Could you check a few things on this model? Use its own coordinates, in mm. A direction names the side the tool comes from. Give positions to 0.01 mm unless a question says otherwise; leave off trailing zeros. Loops run counter-clockwise (first coordinate to the right, second up) from the corner with the lowest first, then second, coordinate; pieces in that order, holes last. Notation, with made-up numbers: (-7, 57.25) -> (42, 57.25) arc R24 cw to (42, 79.25) -> close; hole circle Ø1 at (18, -15). An arc over 180 degrees is marked (long way). Write item = value, one per line. Start each with the question number.
1) On a 3-axis mill with a long thin cutter (end or side, diameter ignored), from which of +Z, -Z, +X, -X, +Y, -Y can I reach the whole of each face in a straight line? I mean faces 4 (the face through (-19, -13, -12.7)), 5 (the face through (123.87, -3.22, -26.05)), 6 (the face through (95, -13, 12.232)). Say none if no direction works.
2) If we mould it in two halves opening along Y, with no side actions, what happens to faces 1 (the face through (82, -13, -38.568)), 2 (the face through (110.886, -18.054, -25.69)), 3 (the face through (123.87, -22.18, 24.75))? For each: +Y half, -Y half, draft (parallel to the pull), parting line (faces both ways), or undercut.
3) I want a section at C-C (y = -21.5). List the corners of the cut face in (x, z) for me, and give its area (3 significant figures).
4) I want a section at A-A (y = -12.7). List the corners of the cut face in (x, z) for me, and give its area (3 significant figures).
5) I need wall thicknesses on probe 1 along Z at (x, y) = (92, -15.5); probe 2 along Y at (x, z) = (114.3, -21); probe 3 along Z at (x, y) = (-38.1, -14.5). Which ranges of each line are inside material? Lowest first, please. Write a range as from..to.
6) I want a section at D-D (x = 114.3). List the corners of the cut face in (y, z) for me.
7) I want a section at B-B (x = -38.1). List the corners of the cut face in (y, z) for me, and give its area (3 significant figures).
8) I'm going to push flat-ended pins straight in: pin 1 Ø8 at (y, z) = (-8, 27.5) entering from -X; pin 2 Ø7.5 at (x, y) = (-25, -13) entering from +Z; pin 3 Ø7.5 at (x, y) = (-21.5, -14) entering from -Z; pin 4 Ø7.5 at (x, y) = (114.3, -12.7) entering from -Z. Where does each tip first touch, or does it pass through?
from build123d import *

# Parameters (mm, degrees)
F0_R     = 6.35
F1_DEPTH = 25.4
F3_D     = 12.7
F4_SIZE  = 6.35


with BuildPart() as f1:
    # F0 (on Front) → F1 (new body)
    with BuildSketch(Plane.XZ):
        with BuildLine():
            Line((12.7, 12.7), (-50.8, 12.7))
            Line((-50.8, 12.7), (-50.8, -12.7))
            Line((-50.8, -12.7), (12.7, -12.7))
            ThreePointArc((12.7, -12.7), (21.680256, -16.419744), (25.4, -25.4))
            Line((25.4, -25.4), (25.4, -25.867894))
            ThreePointArc((25.4, -25.867894), (29.119744, -34.84815), (38.1, -38.567894))
            Line((38.1, -38.567894), (127, -38.567894))
            Line((127, -38.567894), (127, -13.167894))
            Line((127, -13.167894), (63.5, -13.167894))
            ThreePointArc((63.5, -13.167894), (54.519744, -9.44815), (50.8, -0.467894))
            ThreePointArc((50.8, -0.467894), (54.519744, 8.512362), (63.5, 12.232106))
            Line((63.5, 12.232106), (127, 12.232106))
            Line((127, 12.232106), (127, 37.632106))
            Line((127, 37.632106), (38.1, 37.632106))
            ThreePointArc((38.1, 37.632106), (29.119744, 33.912362), (25.4, 24.932106))
            Line((25.4, 24.932106), (25.4, 25.4))
            ThreePointArc((25.4, 25.4), (21.680256, 16.419744), (12.7, 12.7))
        make_face()
        with Locations((-38.1, 0)):
            Circle(F0_R, mode=Mode.SUBTRACT)
    extrude(amount=F1_DEPTH)

    # F3 (through all)
    with Locations(Plane(origin=(0, 0, -38.567894), x_dir=(1, 0, 0), z_dir=(0, 0, -1))):
        with Locations((114.3, 12.7)):
            Hole(F3_D / 2)

    # F4
    f4_edges = [f1.edges().sort_by_distance(p)[0] for p in [
        (127, -25.4, -25.867894),
        (127, 0, -25.867894),
        (127, -25.4, 24.932106),
        (127, 0, 24.932106),
    ]]
    chamfer(f4_edges, length=F4_SIZE)


solid = f1.part
Answer list:
q1.face_4 = -Z, -X, +Y, -Y
q1.face_5 = +Z, -Z, +X, +Y
q1.face_6 = +X, +Y, -Y
q2.face_1 = draft
q2.face_2 = undercut
q2.face_3 = -Y half
q3.outline = (-50.8, -12.7) -> (12.7, -12.7) arc R12.7 cw to (25.4, -25.4) -> (25.4, -25.87) arc R12.7 ccw to (38.1, -38.57) -> (124.55, -38.57) -> (124.55, -13.17) -> (63.5, -13.17) arc R12.7 cw to (63.5, 12.23) -> (124.55, 12.23) -> (124.55, 37.63) -> (38.1, 37.63) arc R12.7 ccw to (25.4, 24.93) -> (25.4, 25.4) arc R12.7 cw to (12.7, 12.7) -> (-50.8, 12.7) -> close; hole circle Ø12.7 at (-38.1, 0)
q3.area = 7,560 mm^2
q4.outline = (-50.8, -12.7) -> (12.7, -12.7) arc R12.7 cw to (25.4, -25.4) -> (25.4, -25.87) arc R12.7 ccw to (38.1, -38.57) -> (107.95, -38.57) -> (107.95, -13.17) -> (63.5, -13.17) arc R12.7 cw to (63.5, 12.23) -> (107.95, 12.23) -> (107.95, 37.63) -> (38.1, 37.63) arc R12.7 ccw to (25.4, 24.93) -> (25.4, 25.4) arc R12.7 cw to (12.7, 12.7) -> (-50.8, 12.7) -> close; (120.65, -38.57) -> (127, -38.57) -> (127, -13.17) -> (120.65, -13.17) -> close; (120.65, 12.23) -> (127, 12.23) -> (127, 37.63) -> (120.65, 37.63) -> close; hole circle Ø12.7 at (-38.1, 0)
q4.area = 7,040 mm^2
q5.probe_1 = -38.57..-13.17, 12.23..37.63
q5.probe_2 = -25.4..-19.05, -6.35..0
q5.probe_3 = -12.7..-6.35, 6.35..12.7
q6.outline = (-25.4, -38.57) -> (-19.05, -38.57) -> (-19.05, -13.17) -> (-25.4, -13.17) -> close; (-25.4, 12.23) -> (-19.05, 12.23) -> (-19.05, 37.63) -> (-25.4, 37.63) -> close; (-6.35, -38.57) -> (0, -38.57) -> (0, -13.17) -> (-6.35, -13.17) -> close; (-6.35, 12.23) -> (0, 12.23) -> (0, 37.63) -> (-6.35, 37.63) -> close
q7.outline = (-25.4, -12.7) -> (0, -12.7) -> (0, -6.35) -> (-25.4, -6.35) -> close; (-25.4, 6.35) -> (0, 6.35) -> (0, 12.7) -> (-25.4, 12.7) -> close
q7.area = 323 mm^2
q8.pin_1 = 25.26
q8.pin_2 = 12.7
q8.pin_3 = -12.7
q8.pin_4 = through
